Verification items for the finished model (mm, model axes). Face numbers are marked on the shaded views. A direction names the side the tool comes from. Round coordinates to 2 decimals unless told otherwise and drop trailing zeros. Write each loop counter-clockwise with the first axis right and the second up, starting at its lowest first coordinate (ties: lowest second). Pieces come first, ordered by that corner, then holes. Notation, with made-up numbers: M 82.5,84.25 L 131.5,84.25 A19 cw 131.5,121.25 Z; hole C 4,-26 d5. An arc over 180 degrees is marked long. One line per question, with ' | ' between items. Start each with the question number.
Q1. Release check for a two-part mould opening along Y. For the marked faces 1, 2, 3 and 4 record: released by +Y, released by -Y, zero draft, split by the parting line, or undercut.
Q2. Thickness scan on line 1 along X through (y, z) = (5, 15.75); line 2 along Y through (x, z) = (-76, 7.25); line 3 along X through (y, z) = (29.5, 1.25). Record the ranges inside material, lowest first. Write a range as from..to.
Q3. Cross-section at B-B (y = 31.5). Record the boundary of the cut face in (x, z) (3 decimals).
Q4. Gauge pin test, flat ends, axial feed: pin 1 (5 mm diameter, centred on x = -88.5, y = 31.5, fed in from +Z) (3 decimals); pin 2 (8 mm diameter, centred on x = 60, y = 29.5, fed in from -Z). Record the tip position at first contact, or that the pin passes through.
Q5. Cross-section at A-A (z = 3). State how many separate pieces and enclosed holes the cut face has, then the cut area to 3 significant figures.
Q6. Cross-section at D-D (x = -24.5). Record the boundary of the cut face in (y, z).
Q7. Cross-section at C-C (x = -80.5). Record the boundary of the cut face in (y, z) (3 decimals), then the cut area to 3 significant figures.
Q8. Tool access check on the marked faces 5 and 6. Record the directions out of +Z, -Z, +X, -X, +Y, -Y that give a thin tool (end or side, any length) a straight path to the whole face; none if there is none.
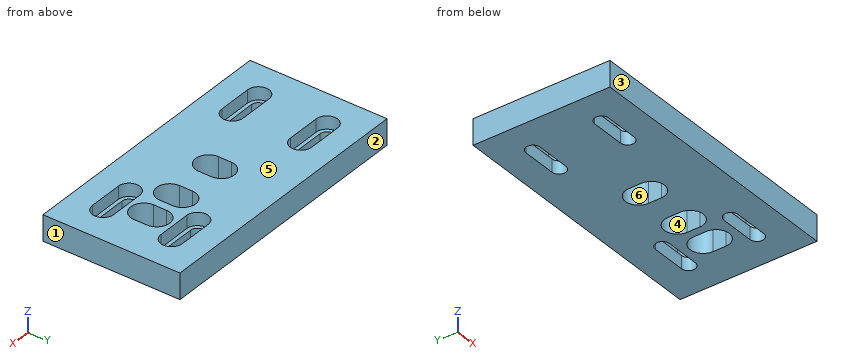
from build123d import *

# Parameters (mm, degrees)
F0_W     = 203.2
F0_H     = 101.6
F1_DEPTH = 19.05
F3_DEPTH = 19.051
F4_DEPTH = 9.525
F6_DEPTH = 19.051


with BuildPart() as f1:
    # F0 (on Top) → F1 (new body)
    with BuildSketch(Plane.XY):
        with Locations((-19.338908, 2.951313)):
            Rectangle(F0_W, F0_H)
    extrude(amount=F1_DEPTH)

    # F2 (on face) → F3 (cut, through all)
    with BuildSketch(Plane.XY.offset(19.05)):
        with BuildLine():
            ThreePointArc((-95.538908, 33.507513), (-100.695108, 28.351313), (-95.538908, 23.195113))
            Line((-95.538908, 23.195113), (-70.138908, 23.195113))
            ThreePointArc((-70.138908, 23.195113), (-64.982708, 28.351313), (-70.138908, 33.507513))
            Line((-70.138908, 33.507513), (-95.538908, 33.507513))
        make_face()
        with BuildLine():
            Line((56.861092, 33.507513), (31.461092, 33.507513))
            ThreePointArc((31.461092, 33.507513), (26.304892, 28.351313), (31.461092, 23.195113))
            Line((31.461092, 23.195113), (56.861092, 23.195113))
            ThreePointArc((56.861092, 23.195113), (62.017292, 28.351313), (56.861092, 33.507513))
        make_face()
        with BuildLine():
            Line((31.461092, -27.604887), (56.861092, -27.604887))
            ThreePointArc((56.861092, -27.604887), (62.017292, -22.448687), (56.861092, -17.292487))
            Line((56.861092, -17.292487), (31.461092, -17.292487))
            ThreePointArc((31.461092, -17.292487), (26.304892, -22.448687), (31.461092, -27.604887))
        make_face()
        with BuildLine():
            Line((-70.138908, -17.292487), (-95.538908, -17.292487))
            ThreePointArc((-95.538908, -17.292487), (-100.695108, -22.448687), (-95.538908, -27.604887))
            Line((-95.538908, -27.604887), (-70.138908, -27.604887))
            ThreePointArc((-70.138908, -27.604887), (-64.982708, -22.448687), (-70.138908, -17.292487))
        make_face()
    extrude(amount=-F3_DEPTH, mode=Mode.SUBTRACT)

    # F2 (on face) → F4 (cut)
    with BuildSketch(Plane.XY.offset(19.05)):
        with BuildLine():
            ThreePointArc((-95.538908, 33.507513), (-100.695108, 28.351313), (-95.538908, 23.195113))
            Line((-95.538908, 23.195113), (-70.138908, 23.195113))
            ThreePointArc((-70.138908, 23.195113), (-64.982708, 28.351313), (-70.138908, 33.507513))
            Line((-70.138908, 33.507513), (-95.538908, 33.507513))
        make_face()
        with BuildLine():
            ThreePointArc((-95.538908, 36.288813), (-103.476408, 28.351313), (-95.538908, 20.413813))
            Line((-95.538908, 20.413813), (-70.138908, 20.413813))
            ThreePointArc((-70.138908, 20.413813), (-62.201408, 28.351313), (-70.138908, 36.288813))
            Line((-70.138908, 36.288813), (-95.538908, 36.288813))
        make_face()
        with BuildLine():
            Line((-70.138908, 23.195113), (-95.538908, 23.195113))
            ThreePointArc((-95.538908, 23.195113), (-100.695108, 28.351313), (-95.538908, 33.507513))
            Line((-95.538908, 33.507513), (-70.138908, 33.507513))
            ThreePointArc((-70.138908, 33.507513), (-64.982708, 28.351313), (-70.138908, 23.195113))
        make_face(mode=Mode.SUBTRACT)
        with BuildLine():
            Line((56.861092, 36.288813), (31.461092, 36.288813))
            ThreePointArc((31.461092, 36.288813), (23.523592, 28.351313), (31.461092, 20.413813))
            Line((31.461092, 20.413813), (56.861092, 20.413813))
            ThreePointArc((56.861092, 20.413813), (64.798592, 28.351313), (56.861092, 36.288813))
        make_face()
        with BuildLine():
            ThreePointArc((31.461092, 23.195113), (26.304892, 28.351313), (31.461092, 33.507513))
            Line((31.461092, 33.507513), (56.861092, 33.507513))
            ThreePointArc((56.861092, 33.507513), (62.017292, 28.351313), (56.861092, 23.195113))
            Line((56.861092, 23.195113), (31.461092, 23.195113))
        make_face(mode=Mode.SUBTRACT)
        with BuildLine():
            Line((-95.538908, -30.386187), (-70.138908, -30.386187))
            ThreePointArc((-70.138908, -30.386187), (-62.201408, -22.448687), (-70.138908, -14.511187))
            Line((-70.138908, -14.511187), (-95.538908, -14.511187))
            ThreePointArc((-95.538908, -14.511187), (-103.476408, -22.448687), (-95.538908, -30.386187))
        make_face()
        with BuildLine():
            ThreePointArc((-95.538908, -27.604887), (-100.695108, -22.448687), (-95.538908, -17.292487))
            Line((-95.538908, -17.292487), (-70.138908, -17.292487))
            ThreePointArc((-70.138908, -17.292487), (-64.982708, -22.448687), (-70.138908, -27.604887))
            Line((-70.138908, -27.604887), (-95.538908, -27.604887))
        make_face(mode=Mode.SUBTRACT)
        with BuildLine():
            Line((31.461092, -30.386187), (56.861092, -30.386187))
            ThreePointArc((56.861092, -30.386187), (64.798592, -22.448687), (56.861092, -14.511187))
            Line((56.861092, -14.511187), (31.461092, -14.511187))
            ThreePointArc((31.461092, -14.511187), (23.523592, -22.448687), (31.461092, -30.386187))
        make_face()
        with BuildLine():
            ThreePointArc((56.861092, -17.292487), (62.017292, -22.448687), (56.861092, -27.604887))
            Line((56.861092, -27.604887), (31.461092, -27.604887))
            ThreePointArc((31.461092, -27.604887), (26.304892, -22.448687), (31.461092, -17.292487))
            Line((31.461092, -17.292487), (56.861092, -17.292487))
        make_face(mode=Mode.SUBTRACT)
    extrude(amount=-F4_DEPTH, mode=Mode.SUBTRACT)

    # F5 (on face) → F6 (cut, through all)
    with BuildSketch(Plane.XY.offset(19.05)):
        with BuildLine():
            Line((-28.990908, 7.713813), (-28.990908, 2.951313))
            Line((-28.990908, 2.951313), (-19.338908, 2.951313))
            Line((-19.338908, 2.951313), (-9.686908, 2.951313))
            Line((-9.686908, 2.951313), (-9.686908, 7.713813))
            ThreePointArc((-9.686908, 7.713813), (-19.338908, 17.365813), (-28.990908, 7.713813))
        make_face()
        with BuildLine():
            Line((-19.338908, 2.951313), (-28.990908, 2.951313))
            Line((-28.990908, 2.951313), (-28.990908, -1.811187))
            ThreePointArc((-28.990908, -1.811187), (-19.338908, -11.463187), (-9.686908, -1.811187))
            Line((-9.686908, -1.811187), (-9.686908, 2.951313))
            Line((-9.686908, 2.951313), (-19.338908, 2.951313))
        make_face()
        with BuildLine():
            Line((9.109092, 7.713813), (9.109092, 2.951313))
            Line((9.109092, 2.951313), (18.761092, 2.951313))
            Line((18.761092, 2.951313), (28.413092, 2.951313))
            Line((28.413092, 2.951313), (28.413092, 7.713813))
            ThreePointArc((28.413092, 7.713813), (18.761092, 17.365813), (9.109092, 7.713813))
        make_face()
        with BuildLine():
            Line((18.761092, 2.951313), (9.109092, 2.951313))
            Line((9.109092, 2.951313), (9.109092, -1.811187))
            ThreePointArc((9.109092, -1.811187), (18.761092, -11.463187), (28.413092, -1.811187))
            Line((28.413092, -1.811187), (28.413092, 2.951313))
            Line((28.413092, 2.951313), (18.761092, 2.951313))
        make_face()
        with BuildLine():
            Line((44.161092, 2.951313), (53.813092, 2.951313))
            Line((53.813092, 2.951313), (53.813092, 7.713813))
            ThreePointArc((53.813092, 7.713813), (44.161092, 17.365813), (34.509092, 7.713813))
            Line((34.509092, 7.713813), (34.509092, 2.951313))
            Line((34.509092, 2.951313), (44.161092, 2.951313))
        make_face()
        with BuildLine():
            Line((53.813092, -1.811187), (53.813092, 2.951313))
            Line((53.813092, 2.951313), (44.161092, 2.951313))
            Line((44.161092, 2.951313), (34.509092, 2.951313))
            Line((34.509092, 2.951313), (34.509092, -1.811187))
            ThreePointArc((34.509092, -1.811187), (44.161092, -11.463187), (53.813092, -1.811187))
        make_face()
    extrude(amount=-F6_DEPTH, mode=Mode.SUBTRACT)


solid = f1.part
Determined:
1) face 1: zero draft | face 2: released by +Y | face 3: released by -Y | face 4: undercut
2) line 1: x = -120.94..-28.99, -9.69..9.11, 28.41..34.51, 53.81..82.26 | line 2: y = -47.85..-27.6, -17.29..23.2, 33.51..53.75 | line 3: x = -120.94..-100.57, -65.11..26.43, 61.89..82.26
3) outline: M -120.939,0 L -99.622,0 L -99.622,9.525 L -102.825,9.525 L -102.825,19.05 L -120.939,19.05 Z; M -66.056,0 L 27.378,0 L 27.378,9.525 L 24.175,9.525 L 24.175,19.05 L -62.853,19.05 L -62.853,9.525 L -66.056,9.525 Z; M 60.944,0 L 82.261,0 L 82.261,19.05 L 64.147,19.05 L 64.147,9.525 L 60.944,9.525 Z
4) pin 1: stops at z = 9.525 | pin 2: stops at z = 0
5) separate pieces: 1 | enclosed holes: 7 | area: 17,800 mm²
6) outline: M -47.85,0 L -9.97,0 L -9.97,19.05 L -47.85,19.05 Z; M 15.87,0 L 53.75,0 L 53.75,19.05 L 15.87,19.05 Z
7) outline: M -47.849,0 L -27.605,0 L -27.605,9.525 L -30.386,9.525 L -30.386,19.05 L -47.849,19.05 Z; M -17.292,0 L 23.195,0 L 23.195,9.525 L 20.414,9.525 L 20.414,19.05 L -14.511,19.05 L -14.511,9.525 L -17.292,9.525 Z; M 33.508,0 L 53.751,0 L 53.751,19.05 L 36.289,19.05 L 36.289,9.525 L 33.508,9.525 Z | area: 1,440 mm²
8) face 5: +Z, +X, -X, +Y, -Y | face 6: +Z, -Z
